```python
from build123d import *

# Parameters (mm, degrees)
TAP_PATTERN_COUNT = 16
CHAMFER1_SIZE     = 2.54
CHAMFER1_SIZE2    = 4.399409051


with BuildPart() as part:
    # Sketch1 → Revolve1 (revolve)
    with BuildSketch(Plane.XY):
        Polygon((0, 0), (-58.4454, 0), (-58.4454, 38.1), (-63.5, 38.1), (-63.5, 63.5), (0, 63.5), align=None)
    revolve(axis=Axis((0, 63.5, 0), (0, -1, 0)))

    # Sketch13 → 1/4-28 Tap (revolve, cut)
    with BuildSketch(Plane(origin=(0, 12.7, 58.4454), x_dir=(0, -1, 0), z_dir=(1, 0, 0))):
        Polygon((0, 0), (0, 20.675388061), (2.7051, 19.05), (2.7051, 0), align=None)
    f_1_4_28_tap = revolve(axis=Axis((0, 12.7, 64.7954), (0, 0, -1)), mode=Mode.SUBTRACT)

    # Tap Pattern: 1/4-28 Tap ×16 about axis
    tap_pattern_axis = Axis((0, 0, 0), (0, 1, 0))
    for i in range(1, TAP_PATTERN_COUNT):
        add(f_1_4_28_tap.rotate(tap_pattern_axis, i * 360 / TAP_PATTERN_COUNT), mode=Mode.SUBTRACT)

    # Chamfer1
    chamfer1_edges = [part.edges().sort_by_distance(p)[0] for p in [
        (58.4454, 0, 0),
    ]]
    chamfer1_side = [part.faces().sort_by_distance(p)[0] for p in [
        (0, 0, 0),
    ]]
    chamfer(chamfer1_edges, length=CHAMFER1_SIZE, length2=CHAMFER1_SIZE2, reference=chamfer1_side[0])


solid = part.part
```
The listing builds one solid part. Answer for the finished solid, in the listing's coordinates (mm). A direction names the side the tool comes from. Round coordinates to 2 decimals unless told otherwise and drop trailing zeros. Loops run counter-clockwise (first coordinate to the right, second up) from the corner with the lowest first, then second, coordinate; pieces in that order, holes last. Notation, with made-up numbers: (-21.75, -25) - (13.25, -25) arc R30 ccw to (13.25, 1) - close; hole circle Ø2 at (50, -36.5). An arc over 180 degrees is marked (long way). Return JSON: item names as keys, results as strings. Group by question number.
1. Consider probe 1 along Y at (x, z) = (-49, 0); probe 2 along X at (y, z) = (11.5, 34.5); probe 3 along X at (y, z) = (11.5, -43). Determine where each line is inside the solid, lowest interval first.
2. The mould has two halves that part along Y. Classify faces 6 (the flat face through (1, 63.5, -1)), 7 (the conical face through (-0.18, 12.27, -38.05)), 8 (the conical face through (-53.48, 0.28, -16.84)): pulls with the +Y half, pulls with the -Y half, needs draft (parallel to the pull), parting line crosses it, or undercut.
3. The part is cut by section A-A on y = 18. Determine the outline of the cut face in (x, z), then the cut area to 3 significant figures.
4. The part is cut by section B-B on x = 32.5. State how many separate pieces and enclosed holes the cut face has, then the cut area to 3 significant figures.
5. Which of the six approach directions +Z, -Z, +X, -X, +Y, -Y give full straight-line access (tool end or side, diameter ignored) to faces 1 (the flat face through (-1, 0, -1)), 2 (the cylindrical face through (-49.054, 15.402, -0.119)), 3 (the cylindrical face through (49.054, 14.847, -1.646)), 4 (the cylindrical face through (58.39, 21.49, -2.57)), 5 (the conical face through (-14.947, 12.483, -34.996))?
6. The part is cut by section D-D on y = 59. Determine the outline of the cut face in (x, z), then the cut area to 3 significant figures.
7. Each of these flat-tipped pins is pushed along its axis until it touches: P1, Ø8.5, axis at x = 0, y = 12.7, coming from the +Z side; P2, Ø6, axis at y = 12.7, z = 0, coming from the +X side; P3, Ø7, axis at y = 12.7, z = 0, coming from the -X side. Where does it stop, or does it pass through?
Resolved:
{
 "1": {"probe 1": "y = 0 to 9.99, 15.41 to 63.5", "probe 2": "x = -47.18 to -37.93, -31.07 to 31.07, 37.93 to 47.18", "probe 3": "x = -39.57 to -20.44, -15.19 to -2.42, 2.42 to 15.19, 20.44 to 39.57"},
 "2": {"face 6": "pulls with the +Y half", "face 7": "undercut", "face 8": "pulls with the -Y half"},
 "3": {"outline": "circle Ø116.89 at (0, 0)", "area": "10,700 mm²"},
 "4": {"separate pieces": "1", "enclosed holes": "2", "area": "6,390 mm²"},
 "5": {"face 1": "+Z, -Z, +X, -X, -Y", "face 2": "-X", "face 3": "+X", "face 4": "-Y", "face 5": "none"},
 "6": {"outline": "circle Ø127 at (0, 0)", "area": "12,700 mm²"},
 "7": {"P1": "stops at z = 58.45", "P2": "stops at x = 58.45", "P3": "stops at x = -58.45"}
}
